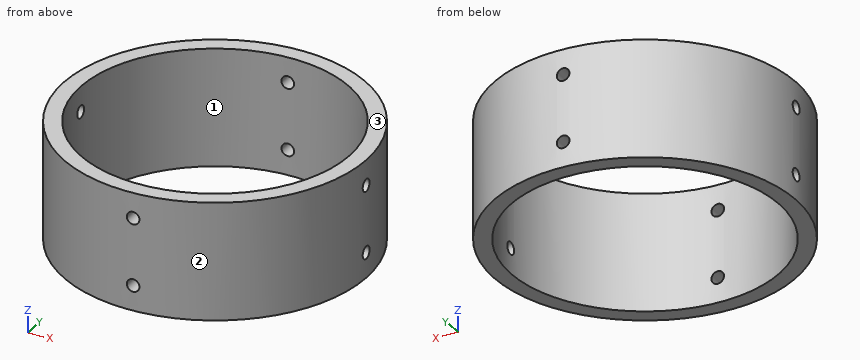
```python
from build123d import *

# Parameters (mm, degrees)
SKETCH1_R           = 18
SKETCH1_R_2         = 16
BOSS_EXTRUDE1_DEPTH = 14
SKETCH2_R           = 0.75
CUT_EXTRUDE1_DEPTH  = 5
CIRPATTERN1_COUNT   = 4


with BuildPart() as part:
    # Sketch1 → Boss-Extrude1 (new body)
    with BuildSketch(Plane.XY):
        Circle(SKETCH1_R)
        Circle(SKETCH1_R_2, mode=Mode.SUBTRACT)
    extrude(amount=BOSS_EXTRUDE1_DEPTH)

    # Sketch2 → Cut-Extrude1 (cut)
    with BuildSketch(Plane(origin=(0, 18, 0), x_dir=(1, 0, 0), z_dir=(0, 1, 0))):
        with Locations((0, -3)):
            Circle(SKETCH2_R)
        with Locations((0, -11)):
            Circle(SKETCH2_R)
    cut_extrude1 = extrude(amount=-CUT_EXTRUDE1_DEPTH, mode=Mode.SUBTRACT)

    # CirPattern1: Cut-Extrude1 ×4 about axis
    cirpattern1_axis = Axis((0, 0, 14), (0, 0, 1))
    for i in range(1, CIRPATTERN1_COUNT):
        add(cut_extrude1.rotate(cirpattern1_axis, i * 360 / CIRPATTERN1_COUNT), mode=Mode.SUBTRACT)


solid = part.part
```
Work out the finished part from the listing and answer in its coordinate system (mm). Face numbers are marked on the shaded views. Coordinates: 2 decimals unless noted, no trailing zeros. Write each loop counter-clockwise with the first axis right and the second up, starting at its lowest first coordinate (ties: lowest second). Pieces come first, ordered by that corner, then holes. Notation, with made-up numbers: (82.25, -22.75) - (116.25, -22.75) arc R22 cw to (116.25, -12.75) - close; hole circle Ø9 at (17.25, 61). An arc over 180 degrees is marked (long way). Answer as a JSON object with one key per item and string values.
Q1. Find section A-A (y = 0). Write down the section's boundary in (x, z).
Results list:
{"outline": "(-18, 0) - (-16, 0) - (-16, 2.25) - (-18, 2.25) - close; (-18, 3.75) - (-16, 3.75) - (-16, 10.25) - (-18, 10.25) - close; (-18, 11.75) - (-16, 11.75) - (-16, 14) - (-18, 14) - close; (16, 0) - (18, 0) - (18, 2.25) - (16, 2.25) - close; (16, 3.75) - (18, 3.75) - (18, 10.25) - (16, 10.25) - close; (16, 11.75) - (18, 11.75) - (18, 14) - (16, 14) - close"}
Q2. Find section C-C (z = 11). Write down the section's boundary in (x, y), plus the area to 3 significant figures.
Results list:
{"outline": "(-17.98, -0.75) arc R18 ccw to (-0.75, -17.98) - (-0.75, -15.98) arc R16 cw to (-15.98, -0.75) - close; (-17.98, 0.75) - (-15.98, 0.75) arc R16 cw to (-0.75, 15.98) - (-0.75, 17.98) arc R18 ccw to start; (0.75, -17.98) arc R18 ccw to (17.98, -0.75) - (15.98, -0.75) arc R16 cw to (0.75, -15.98) - close; (0.75, 15.98) arc R16 cw to (15.98, 0.75) - (17.98, 0.75) arc R18 ccw to (0.75, 17.98) - close", "area": "202 mm^2"}
Q3. For a pull along X with two mould halves and no side action, classify the marked faces 1, 2 and 3 as pulls with the +X half, pulls with the -X half, needs draft (parallel to the pull), parting line crosses it, or undercut.
Results list:
{"face 1": "undercut", "face 2": "parting line crosses it", "face 3": "needs draft"}
Q4. Find section D-D (y = 11.5). Write down the section's boundary in (x, z).
Results list:
{"outline": "(-13.85, 0) - (-11.12, 0) - (-11.12, 14) - (-13.85, 14) - close; (11.12, 0) - (13.85, 0) - (13.85, 14) - (11.12, 14) - close"}
Q5. Consider L1, parallel to Z at x = 0, y = -16.35; L2, parallel to X at y = -7, z = 9.5; L3, parallel to X at y = 3, z = 1.75. Determine where each line is inside the solid, lowest interval first. Write a range as from..to.
Results list:
{"L1": "z = 0..2.25, 3.75..10.25, 11.75..14", "L2": "x = -16.58..-14.39, 14.39..16.58", "L3": "x = -17.75..-15.72, 15.72..17.75"}
Q6. Find section B-B (x = 9). Write down the section's boundary in (y, z).
Results list:
{"outline": "(-15.59, 0) - (-13.23, 0) - (-13.23, 14) - (-15.59, 14) - close; (13.23, 0) - (15.59, 0) - (15.59, 14) - (13.23, 14) - close"}
Q7. Given pin 1 Ø1.4 at (x, z) = (0, 11) entering from +Y; pin 2 Ø2 at (x, z) = (0, 3) entering from +Y; pin 3 Ø6 at (y, z) = (-5, 2) entering from +X; pin 4 Ø2 at (x, z) = (-3, 1.5) entering from +Y, each flat-ended and moving along its own axis, determine where each tip first touches the part or whether it passes through.
Results list:
{"pin 1": "passes through", "pin 2": "stops at y = 18", "pin 3": "stops at x = 17.89", "pin 4": "stops at y = 17.89"}
